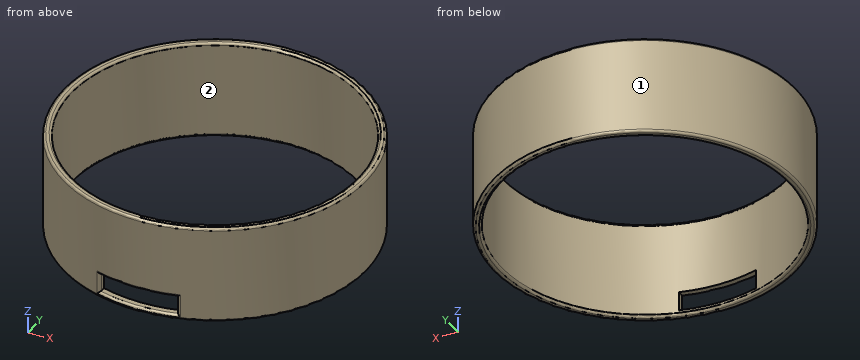
```python
from build123d import *

# Parameters (mm, degrees)
F0_R         = 316.25
F1_DEPTH     = 205.7
F2_R         = 300
F3_DEPTH     = 631
F5_W         = 160
F5_H         = 40
F6_DEPTH     = 796.1248755455
F7_T1_DEPTH  = 40
F7_T10_ANGLE = 33.8359646931
F7_T16_ANGLE = 33.8359646931
F7_T27_ANGLE = 33.8359646931
F7_T31_DEPTH = 56.5905669687
F7_T38_DEPTH = 56.399324286
F7_T42_ANGLE = 33.8359646931
F7_T49_ANGLE = 33.8359646931
F7_T53_DEPTH = 56.5905669687
F7_T60_ANGLE = 33.8359646931
F7_T64_DEPTH = 56.399324286


# Not quite as in the source:
# - a fillet or chamfer that OpenCascade refuses, or shapes differently, is made with other operations: its cross-section is extruded or revolved along the edge and cut away or added


with BuildPart() as f1:
    # F0 (on Top) → F1 (new body)
    with BuildSketch(Plane.XY):
        Circle(F0_R)
    extrude(amount=F1_DEPTH)

    # F2 (on face) → F3 (cut)
    with BuildSketch(Plane.XY.offset(205.7)):
        Circle(F2_R)
    extrude(amount=-F3_DEPTH, mode=Mode.SUBTRACT)

    # F5 (on offset) → F6 (cut)
    with BuildSketch(Plane.XZ.offset(645.5422639847)):
        with Locations((1.6928017139, 30.4630875368)):
            Rectangle(F5_W, F5_H)
    extrude(amount=-F6_DEPTH, mode=Mode.SUBTRACT)

    # F7: fillet of radius 5 on 8 edges, made by hand

    # F7_s2 → F7_t1 (cut)
    with BuildSketch(Plane.XY.offset(10.4630875368)):
        with BuildLine():
            ThreePointArc((88.0854571632, -303.7351061968), (83.6897430437, -302.9306742994), (81.6928017139, -298.9329701304))
            Line((81.6928017139, -298.9329701304), (81.6928017139, -305.5165276186))
            ThreePointArc((81.6928017139, -305.5165276186), (84.8938022614, -304.6425853974), (88.0854571632, -303.7351061968))
        make_face()
        with BuildLine():
            ThreePointArc((-84.6454665316, -304.7116792899), (-80.2815860528, -303.8747654151), (-78.3071982861, -299.8941033327))
            Line((-78.3071982861, -299.8941033327), (-78.3071982861, -306.401770877))
            ThreePointArc((-78.3071982861, -306.401770877), (-81.4807145599, -305.5731592513), (-84.6454665316, -304.7116792899))
        make_face()
    extrude(amount=F7_T1_DEPTH, mode=Mode.SUBTRACT)

    # F7_s3 → F7_t4 (revolve, cut)
    with BuildSketch(Plane.XZ):
        with BuildLine():
            ThreePointArc((316.25, 200.7), (314.7855339059, 204.2355339059), (311.25, 205.7))
            Line((311.25, 205.7), (316.25, 205.7))
            Line((316.25, 205.7), (316.25, 200.7))
        make_face()
    revolve(axis=Axis((0, 0, 205.7), (0, 0, 1)), mode=Mode.SUBTRACT)

    # F7_s5 → F7_t6 (revolve, cut)
    with BuildSketch(Plane.XZ):
        with BuildLine():
            ThreePointArc((305, 205.7), (301.4644660941, 204.2355339059), (300, 200.7))
            Line((300, 200.7), (300, 205.7))
            Line((300, 205.7), (305, 205.7))
        make_face()
    revolve(axis=Axis((0, 0, 205.7), (0, 0, 1)), mode=Mode.SUBTRACT)


with BuildPart() as f7_tool8:
    # F7_s9 → F7_t10 (revolve)
    with BuildSketch(Plane(origin=(0, 0, 0), x_dir=(0, 0, 1), z_dir=(0.9550976314, 0.2962912662, 0))):
        with BuildLine():
            ThreePointArc((55.4630875368, 316.25), (51.9275536309, 314.7855339059), (50.4630875368, 311.25))
            Line((50.4630875368, 311.25), (50.4630875368, 316.25))
            Line((50.4630875368, 316.25), (55.4630875368, 316.25))
        make_face()
    revolve(axis=Axis((0, 0, 50.4630875368), (0, 0, -1)), revolution_arc=F7_T10_ANGLE)

    split(bisect_by=Plane.YZ.offset(-78.3071982861), keep=Keep.TOP)

    split(bisect_by=Plane.YZ.offset(81.6928017139), keep=Keep.BOTTOM)


with BuildPart() as f1_1:
    add(f1.part)

    # F7_t7: cut F7_tool8
    add(f7_tool8.part, mode=Mode.SUBTRACT)


with BuildPart() as f7_tool14:
    # F7_s15 → F7_t16 (revolve)
    with BuildSketch(Plane(origin=(0, 0, 0), x_dir=(0, 0, 1), z_dir=(0.9550976314, 0.2962912662, 0))):
        with BuildLine():
            ThreePointArc((5.4630875368, 316.25), (8.9986214427, 314.7855339059), (10.4630875368, 311.25))
            Line((10.4630875368, 311.25), (10.4630875368, 316.25))
            Line((10.4630875368, 316.25), (5.4630875368, 316.25))
        make_face()
    revolve(axis=Axis((0, 0, 10.4630875368), (0, 0, -1)), revolution_arc=F7_T16_ANGLE)

    split(bisect_by=Plane.YZ.offset(81.6928017139), keep=Keep.BOTTOM)

    split(bisect_by=Plane.YZ.offset(-78.3071982861), keep=Keep.TOP)


with BuildPart() as f1_2:
    add(f1_1.part)

    # F7_t13: cut F7_tool14
    add(f7_tool14.part, mode=Mode.SUBTRACT)

    # F7_s19 → F7_t20 (revolve, cut)
    with BuildSketch(Plane.XZ):
        with BuildLine():
            ThreePointArc((316.25, 5), (314.7855339059, 1.4644660941), (311.25, 0))
            Line((311.25, 0), (316.25, 0))
            Line((316.25, 0), (316.25, 5))
        make_face()
    revolve(axis=Axis((0, 0, 0), (0, 0, 1)), mode=Mode.SUBTRACT)

    # F7_s21 → F7_t22 (revolve, cut)
    with BuildSketch(Plane.XZ):
        with BuildLine():
            ThreePointArc((305, 0), (301.4644660941, 1.4644660941), (300, 5))
            Line((300, 5), (300, 0))
            Line((300, 0), (305, 0))
        make_face()
    revolve(axis=Axis((0, 0, 0), (0, 0, 1)), mode=Mode.SUBTRACT)


with BuildPart() as f7_tool25:
    # F7_s26 → F7_t27 (revolve)
    with BuildSketch(Plane(origin=(0, 0, 0), x_dir=(0, 0, 1), z_dir=(0.9550976314, 0.2962912662, 0))):
        with BuildLine():
            ThreePointArc((55.4630875368, 316.25), (51.9275536309, 314.7855339059), (50.4630875368, 311.25))
            Line((50.4630875368, 311.25), (50.4630875368, 316.25))
            Line((50.4630875368, 316.25), (55.4630875368, 316.25))
        make_face()
    revolve(axis=Axis((0, 0, 50.4630875368), (0, 0, -1)), revolution_arc=F7_T27_ANGLE)

    split(bisect_by=Plane.YZ.offset(81.6928017139), keep=Keep.TOP)


with BuildPart() as f7_tool29:
    # F7_s30 → F7_t31 (new body)
    with BuildSketch(Plane.XY.offset(67.0536545055)):
        with BuildLine():
            ThreePointArc((88.0854571632, -303.7351061968), (83.6897430437, -302.9306742994), (81.6928017139, -298.9329701304))
            Line((81.6928017139, -298.9329701304), (81.6928017139, -305.5165276186))
            ThreePointArc((81.6928017139, -305.5165276186), (84.8938022614, -304.6425853974), (88.0854571632, -303.7351061968))
        make_face()
    extrude(amount=-F7_T31_DEPTH)

    split(bisect_by=Plane.XY.offset(50.4630875368), keep=Keep.TOP)


with BuildPart() as f7_tool25_1:
    add(f7_tool25.part)

    # F7_t33: intersect F7_tool29
    add(f7_tool29.part, mode=Mode.INTERSECT)


with BuildPart() as f1_3:
    add(f1_2.part)

    # F7_t23: cut F7_tool25
    add(f7_tool25_1.part, mode=Mode.SUBTRACT)


with BuildPart() as f7_tool36:
    # F7_s37 → F7_t38 (new body)
    with BuildSketch(Plane.XY.offset(66.8624118228)):
        with BuildLine():
            ThreePointArc((-84.6454665316, -304.7116792899), (-80.2815860528, -303.8747654151), (-78.3071982861, -299.8941033327))
            Line((-78.3071982861, -299.8941033327), (-78.3071982861, -306.401770877))
            ThreePointArc((-78.3071982861, -306.401770877), (-81.4807145599, -305.5731592513), (-84.6454665316, -304.7116792899))
        make_face()
    extrude(amount=-F7_T38_DEPTH)

    split(bisect_by=Plane.XY.offset(50.4630875368), keep=Keep.TOP)


with BuildPart() as f7_tool40:
    # F7_s41 → F7_t42 (revolve)
    with BuildSketch(Plane(origin=(0, 0, 0), x_dir=(0, 0, 1), z_dir=(0.9550976314, 0.2962912662, 0))):
        with BuildLine():
            ThreePointArc((55.4630875368, 316.25), (51.9275536309, 314.7855339059), (50.4630875368, 311.25))
            Line((50.4630875368, 311.25), (50.4630875368, 316.25))
            Line((50.4630875368, 316.25), (55.4630875368, 316.25))
        make_face()
    revolve(axis=Axis((0, 0, 50.4630875368), (0, 0, -1)), revolution_arc=F7_T42_ANGLE)

    split(bisect_by=Plane.YZ.offset(-78.3071982861), keep=Keep.BOTTOM)


with BuildPart() as f7_tool36_1:
    add(f7_tool36.part)

    # F7_t44: intersect F7_tool40
    add(f7_tool40.part, mode=Mode.INTERSECT)


with BuildPart() as f1_4:
    add(f1_3.part)

    # F7_t34: cut F7_tool36
    add(f7_tool36_1.part, mode=Mode.SUBTRACT)


with BuildPart() as f7_tool47:
    # F7_s48 → F7_t49 (revolve)
    with BuildSketch(Plane(origin=(0, 0, 0), x_dir=(0, 0, 1), z_dir=(0.9550976314, 0.2962912662, 0))):
        with BuildLine():
            ThreePointArc((5.4630875368, 316.25), (8.9986214427, 314.7855339059), (10.4630875368, 311.25))
            Line((10.4630875368, 311.25), (10.4630875368, 316.25))
            Line((10.4630875368, 316.25), (5.4630875368, 316.25))
        make_face()
    revolve(axis=Axis((0, 0, 10.4630875368), (0, 0, -1)), revolution_arc=F7_T49_ANGLE)

    split(bisect_by=Plane.YZ.offset(81.6928017139), keep=Keep.TOP)


with BuildPart() as f7_tool51:
    # F7_s52 → F7_t53 (new body)
    with BuildSketch(Plane.XY.offset(50.4630875368)):
        with BuildLine():
            ThreePointArc((88.0854571632, -303.7351061968), (83.6897430437, -302.9306742994), (81.6928017139, -298.9329701304))
            Line((81.6928017139, -298.9329701304), (81.6928017139, -305.5165276186))
            ThreePointArc((81.6928017139, -305.5165276186), (84.8938022614, -304.6425853974), (88.0854571632, -303.7351061968))
        make_face()
    extrude(amount=-F7_T53_DEPTH)

    split(bisect_by=Plane.XY.offset(10.4630875368), keep=Keep.BOTTOM)


with BuildPart() as f7_tool47_1:
    add(f7_tool47.part)

    # F7_t55: intersect F7_tool51
    add(f7_tool51.part, mode=Mode.INTERSECT)


with BuildPart() as f1_5:
    add(f1_4.part)

    # F7_t45: cut F7_tool47
    add(f7_tool47_1.part, mode=Mode.SUBTRACT)


with BuildPart() as f7_tool58:
    # F7_s59 → F7_t60 (revolve)
    with BuildSketch(Plane(origin=(0, 0, 0), x_dir=(0, 0, 1), z_dir=(0.9550976314, 0.2962912662, 0))):
        with BuildLine():
            ThreePointArc((5.4630875368, 316.25), (8.9986214427, 314.7855339059), (10.4630875368, 311.25))
            Line((10.4630875368, 311.25), (10.4630875368, 316.25))
            Line((10.4630875368, 316.25), (5.4630875368, 316.25))
        make_face()
    revolve(axis=Axis((0, 0, 10.4630875368), (0, 0, -1)), revolution_arc=F7_T60_ANGLE)

    split(bisect_by=Plane.YZ.offset(-78.3071982861), keep=Keep.BOTTOM)


with BuildPart() as f7_tool62:
    # F7_s63 → F7_t64 (new body)
    with BuildSketch(Plane.XY.offset(50.4630875368)):
        with BuildLine():
            ThreePointArc((-84.6454665316, -304.7116792899), (-80.2815860528, -303.8747654151), (-78.3071982861, -299.8941033327))
            Line((-78.3071982861, -299.8941033327), (-78.3071982861, -306.401770877))
            ThreePointArc((-78.3071982861, -306.401770877), (-81.4807145599, -305.5731592513), (-84.6454665316, -304.7116792899))
        make_face()
    extrude(amount=-F7_T64_DEPTH)

    split(bisect_by=Plane.XY.offset(10.4630875368), keep=Keep.BOTTOM)


with BuildPart() as f7_tool58_1:
    add(f7_tool58.part)

    # F7_t66: intersect F7_tool62
    add(f7_tool62.part, mode=Mode.INTERSECT)


with BuildPart() as f1_6:
    add(f1_5.part)

    # F7_t56: cut F7_tool58
    add(f7_tool58_1.part, mode=Mode.SUBTRACT)


solid = f1_6.part
```
For this review, take the finished solid that the model builds, in its own axes (mm). Face numbers are marked on the shaded views. Give positions to 0.01 mm unless a question says otherwise; leave off trailing zeros. Order: outer loops, then holes, each group sorted by start corner. A loop starts at its lowest first (then second) coordinate and runs counter-clockwise, first axis right, second up.
1) Take a section at A-A (y = 0). Give the boundary of the cut face in (x, z), then the cut area to 3 significant figures.
2) Insertion check: pin 1 (1.5 mm diameter, centred on y = 121, z = 27, fed in from -X); pin 2 (1 mm diameter, centred on x = -203, z = 136.5, fed in from +Y); pin 3 (3 mm diameter, centred on y = -291.5, z = 29, fed in from -X); pin 4 (11.5 mm diameter, centred on x = -17, y = -304, fed in from -Z). Each pin has a flat end and moves straight along its axis. Give the tip position at first contact, or say it passes through.
3) The part is to be moulded in two halves that separate along Y. For the marked faces 1 and 2, say which applies: released by +Y, released by -Y, zero draft, split by the parting line, or undercut.
4) Wall thickness on line 1 (Y direction, x = 0, z = 76); line 2 (Y direction, x = -233.5, z = 170); line 3 (X direction, y = -154, z = 119.5): over which ranges is each line inside the solid? List them lowest first.
5) Take a section at C-C (z = 126.5). Give the boundary of the cut face in (x, y), then the cut area to 3 significant figures.
6) Take a section at B-B (x = 0). Give the boundary of the cut face in (y, z), then the cut area to 3 significant figures.
7) Take a section at D-D (x = 71). State how many separate pieces and enclosed holes the cut face has, then the cut area to 3 significant figures.
Derived:
1. outline: (-316.25, 5) arc R5 ccw to (-311.25, 0) - (-305, 0) arc R5 ccw to (-300, 5) - (-300, 200.7) arc R5 ccw to (-305, 205.7) - (-311.25, 205.7) arc R5 ccw to (-316.25, 200.7) - close; (300, 5) arc R5 ccw to (305, 0) - (311.25, 0) arc R5 ccw to (316.25, 5) - (316.25, 200.7) arc R5 ccw to (311.25, 205.7) - (305, 205.7) arc R5 ccw to (300, 200.7) - close
1. area: 6,640 mm2
2. pin 1: stops at x = -292.5
2. pin 2: stops at y = 242.92
2. pin 3: stops at x = -126.15
2. pin 4: stops at z = 0
3. face 1: split by the parting line
3. face 2: undercut
4. line 1: y = -316.25 to -300, 300 to 316.25
4. line 2: y = -213.29 to -188.36, 188.36 to 213.29
4. line 3: x = -276.22 to -257.46, 257.46 to 276.22
5. outline: circle Ø632.5 at (0, 0); hole circle Ø600 at (0, 0)
5. area: 31,500 mm2
6. outline: (-316.25, 5) arc R5 ccw to (-311.25, 0) - (-305, 0) arc R5 ccw to (-300, 5) - (-300, 10.46) - (-311.25, 10.46) arc R5 ccw to (-316.25, 5.46) - close; (-316.25, 55.46) arc R5 ccw to (-311.25, 50.46) - (-300, 50.46) - (-300, 200.7) arc R5 ccw to (-305, 205.7) - (-311.25, 205.7) arc R5 ccw to (-316.25, 200.7) - close; (300, 5) arc R5 ccw to (305, 0) - (311.25, 0) arc R5 ccw to (316.25, 5) - (316.25, 200.7) arc R5 ccw to (311.25, 205.7) - (305, 205.7) arc R5 ccw to (300, 200.7) - close
6. area: 5,980 mm2
7. separate pieces: 3
7. enclosed holes: 0
7. area: 6,150 mm2
